Design review of the part built by this model. Coordinates are the model's own, in mm. Coordinates: 2 decimals unless noted, no trailing zeros. Loops run counter-clockwise (first coordinate to the right, second up) from the corner with the lowest first, then second, coordinate; pieces in that order, holes last. Notation, with made-up numbers: (-39.75, 82.25) -> (-30.75, 82.25) arc R19 cw to (-30.75, 95.25) -> close; hole circle Ø11 at (-29, 22.5). An arc over 180 degrees is marked (long way). Answer as a JSON object with one key per item and string values.
```python
from build123d import *

# Parameters (mm, degrees)
CROQUIS1_R              = 1.55
SALIENTE_EXTRUIR1_DEPTH = 21
CROQUIS2_R              = 0.4
SALIENTE_EXTRUIR2_DEPTH = 6
CROQUIS3_R              = 0.5
CROQUIS3_R_2            = 0.4
SALIENTE_EXTRUIR3_DEPTH = 1
REDONDEO1_R             = 0.5


with BuildPart() as part:
    # Croquis1 → Saliente-Extruir1 (new body)
    with BuildSketch(Plane.XY):
        Circle(CROQUIS1_R)
    extrude(amount=SALIENTE_EXTRUIR1_DEPTH)

    # Croquis2 → Saliente-Extruir2 (add)
    with BuildSketch(Plane.XY.offset(21)):
        with Locations((0.75, 0)):
            Circle(CROQUIS2_R)
        with Locations((-0.75, 0)):
            Circle(CROQUIS2_R)
    extrude(amount=SALIENTE_EXTRUIR2_DEPTH)

    # Croquis3 → Saliente-Extruir3 (add)
    with BuildSketch(Plane.XY.offset(21)):
        with Locations((-0.75, 0)):
            Circle(CROQUIS3_R)
        with Locations((-0.75, 0)):
            Circle(CROQUIS3_R_2, mode=Mode.SUBTRACT)
        with Locations((0.75, 0)):
            Circle(CROQUIS3_R)
        with Locations((0.75, 0)):
            Circle(CROQUIS3_R_2, mode=Mode.SUBTRACT)
    extrude(amount=SALIENTE_EXTRUIR3_DEPTH)

    # Redondeo1
    redondeo1_edges = [part.edges().sort_by_distance(p)[0] for p in [
        (-1.55, 0, 0),
    ]]
    fillet(redondeo1_edges, radius=REDONDEO1_R)


solid = part.part
```
1) Add section A-A, the plane z = 21.25. Give the boundary of the cut face in (x, y), and give its area (3 significant figures).
Completed:
{"outline": "circle Ø1 at (-0.75, 0); circle Ø1 at (0.75, 0)", "area": "1.57 mm²"}
2) Add section D-D, the plane z = 3.25. Give the boundary of the cut face in (x, y), and give its area (3 significant figures).
Completed:
{"outline": "circle Ø3.1 at (0, 0)", "area": "7.55 mm²"}
3) Add section B-B, the plane y = 0. Give the boundary of the cut face in (x, z), and give its area (3 significant figures).
Completed:
{"outline": "(-1.55, 0.5) arc R0.5 ccw to (-1.05, 0) -> (1.05, 0) arc R0.5 ccw to (1.55, 0.5) -> (1.55, 21) -> (1.25, 21) -> (1.25, 22) -> (1.15, 22) -> (1.15, 27) -> (0.35, 27) -> (0.35, 22) -> (0.25, 22) -> (0.25, 21) -> (-0.25, 21) -> (-0.25, 22) -> (-0.35, 22) -> (-0.35, 27) -> (-1.15, 27) -> (-1.15, 22) -> (-1.25, 22) -> (-1.25, 21) -> (-1.55, 21) -> close", "area": "75.0 mm²"}
4) The part is to be moulded in two halves that separate along X. For faces 1 (the cylindrical face through (0.715, -1.375, 10.606)), 2 (the cylindrical face through (-0.858, -0.488, 21.493)), 3 (the flat face through (0, 0, 0)), say which applies: pulls with the +X half, pulls with the -X half, needs draft (parallel to the pull), parting line crosses it, or undercut.
Completed:
{"face 1": "parting line crosses it", "face 2": "undercut", "face 3": "needs draft"}
5) Add section C-C, the plane x = 0. Give the boundary of the cut face in (y, z).
Completed:
{"outline": "(-1.55, 0.5) arc R0.5 ccw to (-1.05, 0) -> (1.05, 0) arc R0.5 ccw to (1.55, 0.5) -> (1.55, 21) -> (-1.55, 21) -> close"}
6) Wall thickness on probe 1 along Z at (x, y) = (-0.2, -0.1); probe 2 along Y at (x, z) = (0.1, 10); probe 3 along X at (y, z) = (-0.2, 22.5): over which ranges is each line inside the solid? List them lowest first.
Completed:
{"probe 1": "0 to 21", "probe 2": "-1.55 to 1.55", "probe 3": "-1.1 to -0.4, 0.4 to 1.1"}
